Geometry check sheet. Reference: the model listing, model coordinates, mm. Give positions to 0.01 mm unless a question says otherwise; leave off trailing zeros. Write each loop counter-clockwise with the first axis right and the second up, starting at its lowest first coordinate (ties: lowest second). Pieces come first, ordered by that corner, then holes. Notation, with made-up numbers: (-22.75, -0.5) -> (28.25, -0.5) arc R16 ccw to (28.25, 15.5) -> close; hole circle Ø9 at (8, 40.5). An arc over 180 degrees is marked (long way). Write item = value, one per line. Start each with the question number.
1. Depth check by flat-ended pin: P1, Ø6, axis at x = -72.07, y = -115.97, coming from the -Z side; P2, Ø2.5, axis at x = 67.42, y = 66.68, coming from the -Z side; P3, Ø1.2, axis at y = -100.5, z = 44.5, coming from the -X side. Enter the tip coordinate at first touch or a pass-through.
2. Thickness scan on line 1 along Y through (x, z) = (16.5, 43.9) (3 decimals); line 2 along X through (y, z) = (115, 44.25); line 3 along X through (y, z) = (-67.5, 44.95). Record the ranges inside material, lowest first.
3. Cross-section at C-C, the plane z = 44.15. State how many separate pieces and enclosed holes the cut face has, plus the area to 3 significant figures.
4. Cross-section at A-A, the plane y = -13. Record the cut outline in (x, z).
5. Cross-section at D-D, the plane y = -44. Record the cut outline in (x, z), plus the area to 3 significant figures.
6. Cross-section at B-B, the plane x = -131. Record the cut outline in (y, z).
```python
from build123d import *

# Parameters (mm, degrees)
SKETCH_R        = 2.3622
SKETCH_R_2      = 17.78
PAD_DEPTH       = 2.3622
FILLET_R        = 6.35
FILLET001_R     = 6.35
FILLET002_R     = 6.35
FILLET003_R     = 6.35
FILLET004_R     = 6.35
FILLET005_R     = 3.175
FILLET006_R     = 3.175
FILLET007_R     = 6.35
FILLET008_R     = 6.35
FILLET009_R     = 6.35
FILLET010_R     = 6.35
FILLET011_R     = 6.35
FILLET012_R     = 3.175
FILLET013_R     = 3.175
SKETCH001_R     = 4.79425
POCKET_DEPTH    = 2.3632
SKETCH002_R     = 2.2479
POCKET001_DEPTH = 2.3632
SKETCH003_R     = 2.2479
POCKET002_DEPTH = 4.99999


with BuildPart() as part:
    # Sketch (on DatumPlane) → Pad (new body)
    with BuildSketch(Plane.XY.offset(43.6758)):
        Polygon((40.4368, 73.025), (-40.4368, 73.025), (-40.4368, 127), (-65.8368, 127), (-197.6882, 22.225), (-197.6882, -22.225), (-65.8368, -127), (-40.4368, -127), (-40.4368, -73.025), (40.4368, -73.025), (40.4368, -127), (72.1868, -127), (72.1868, 127), (40.4368, 127), align=None)
        with Locations((-21.3868, 66.675)):
            Circle(SKETCH_R, mode=Mode.SUBTRACT)
        with Locations((-21.3868, 53.975)):
            Circle(SKETCH_R, mode=Mode.SUBTRACT)
        with Locations((-21.3868, -53.975)):
            Circle(SKETCH_R, mode=Mode.SUBTRACT)
        with Locations((-21.3868, -66.675)):
            Circle(SKETCH_R, mode=Mode.SUBTRACT)
        with Locations((15.0368, 66.675)):
            Circle(SKETCH_R, mode=Mode.SUBTRACT)
        with Locations((15.24, 53.975)):
            Circle(SKETCH_R, mode=Mode.SUBTRACT)
        with Locations((15.24, -53.975)):
            Circle(SKETCH_R, mode=Mode.SUBTRACT)
        with Locations((15.24, -66.675)):
            Circle(SKETCH_R, mode=Mode.SUBTRACT)
        with Locations((-165.9382, 0)):
            Circle(SKETCH_R_2, mode=Mode.SUBTRACT)
    extrude(amount=PAD_DEPTH)

    # Fillet
    fillet_edges = [part.edges().sort_by_distance(p)[0] for p in [
        (-197.6882, -22.225, 44.8569),
    ]]
    fillet(fillet_edges, radius=FILLET_R)

    # Fillet001
    fillet001_edges = [part.edges().sort_by_distance(p)[0] for p in [
        (-65.8368, -127, 44.8569),
    ]]
    fillet(fillet001_edges, radius=FILLET001_R)

    # Fillet002
    fillet002_edges = [part.edges().sort_by_distance(p)[0] for p in [
        (-40.4368, -127, 44.8569),
    ]]
    fillet(fillet002_edges, radius=FILLET002_R)

    # Fillet003
    fillet003_edges = [part.edges().sort_by_distance(p)[0] for p in [
        (-40.4368, -73.025, 44.8569),
    ]]
    fillet(fillet003_edges, radius=FILLET003_R)

    # Fillet004
    fillet004_edges = [part.edges().sort_by_distance(p)[0] for p in [
        (40.4368, -73.025, 44.8569),
    ]]
    fillet(fillet004_edges, radius=FILLET004_R)

    # Fillet005
    fillet005_edges = [part.edges().sort_by_distance(p)[0] for p in [
        (40.4368, -127, 44.8569),
    ]]
    fillet(fillet005_edges, radius=FILLET005_R)

    # Fillet006
    fillet006_edges = [part.edges().sort_by_distance(p)[0] for p in [
        (72.1868, -127, 44.8569),
    ]]
    fillet(fillet006_edges, radius=FILLET006_R)

    # Fillet007
    fillet007_edges = [part.edges().sort_by_distance(p)[0] for p in [
        (-197.6882, 22.225, 44.8569),
    ]]
    fillet(fillet007_edges, radius=FILLET007_R)

    # Fillet008
    fillet008_edges = [part.edges().sort_by_distance(p)[0] for p in [
        (-65.8368, 127, 44.8569),
    ]]
    fillet(fillet008_edges, radius=FILLET008_R)

    # Fillet009
    fillet009_edges = [part.edges().sort_by_distance(p)[0] for p in [
        (-40.4368, 127, 44.8569),
    ]]
    fillet(fillet009_edges, radius=FILLET009_R)

    # Fillet010
    fillet010_edges = [part.edges().sort_by_distance(p)[0] for p in [
        (40.4368, 73.025, 44.8569),
    ]]
    fillet(fillet010_edges, radius=FILLET010_R)

    # Fillet011
    fillet011_edges = [part.edges().sort_by_distance(p)[0] for p in [
        (-40.4368, 73.025, 44.8569),
    ]]
    fillet(fillet011_edges, radius=FILLET011_R)

    # Fillet012
    fillet012_edges = [part.edges().sort_by_distance(p)[0] for p in [
        (40.4368, 127, 44.8569),
    ]]
    fillet(fillet012_edges, radius=FILLET012_R)

    # Fillet013
    fillet013_edges = [part.edges().sort_by_distance(p)[0] for p in [
        (72.1868, 127, 44.8569),
    ]]
    fillet(fillet013_edges, radius=FILLET013_R)

    # Sketch001 (on Face39 of Fillet013) → Pocket (cut, through all)
    with BuildSketch(Plane.XY.offset(46.038)):
        with Locations((-26.2382, 0)):
            Circle(SKETCH001_R)
    extrude(amount=-POCKET_DEPTH, mode=Mode.SUBTRACT)

    # Sketch002 (on Face44 of Pocket) → Pocket001 (cut, through all)
    with BuildSketch(Plane.XY.offset(46.038)):
        with Locations((-96.923253, -96.214243)):
            Circle(SKETCH002_R)
        with Locations((-72.065864, -115.967033)):
            Circle(SKETCH002_R)
        with Locations((-72.065864, 115.967033)):
            Circle(SKETCH002_R)
        with Locations((-96.923253, 96.214243)):
            Circle(SKETCH002_R)
    extrude(amount=-POCKET001_DEPTH, mode=Mode.SUBTRACT)

    # Sketch003 (on Face48 of Pocket001) → Pocket002 (cut)
    with BuildSketch(Plane.XY.offset(46.038)):
        with Locations((67.4243, -117.475)):
            Circle(SKETCH003_R)
        with Locations((67.4243, -66.675)):
            Circle(SKETCH003_R)
        with Locations((67.4243, 117.475)):
            Circle(SKETCH003_R)
        with Locations((67.4243, 66.675)):
            Circle(SKETCH003_R)
        with Locations((-177.3809, 19.819338)):
            Circle(SKETCH003_R)
        with Locations((-177.3809, -19.819338)):
            Circle(SKETCH003_R)
        with Locations((-143.0528, 0)):
            Circle(SKETCH003_R)
    extrude(amount=-POCKET002_DEPTH, mode=Mode.SUBTRACT)


solid = part.part
```
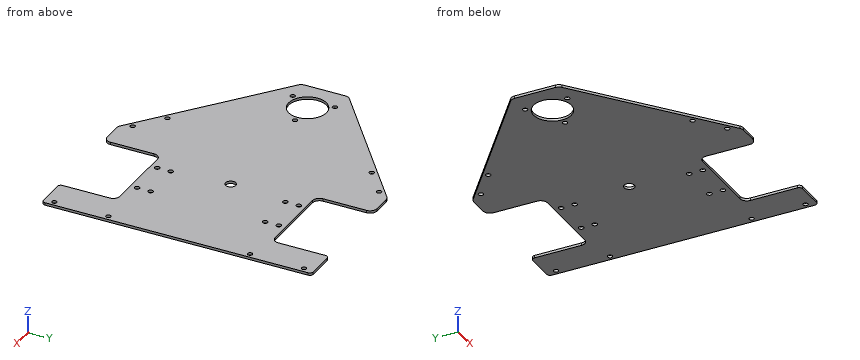
Answers:
q1.P1 = 43.68
q1.P2 = through
q1.P3 = -99.94
q2.line_1 = -73.025 to -68.673, -64.677 to -55.973, -51.977 to 51.977, 55.973 to 64.821, 68.529 to 73.025
q2.line_2 = -80.94 to -74.1, -70.04 to -40.44, 40.44 to 72.19
q2.line_3 = -140.71 to -23.6, -19.17 to 13.03, 17.45 to 65.33, 69.52 to 72.19
q3.separate_pieces = 1
q3.enclosed_holes = 21
q3.area = 44,600 mm^2
q4.outline = (-197.69, 43.68) -> (-178.07, 43.68) -> (-178.07, 46.04) -> (-197.69, 46.04) -> close; (-153.81, 43.68) -> (72.19, 43.68) -> (72.19, 46.04) -> (-153.81, 46.04) -> close
q5.outline = (-170.29, 43.68) -> (72.19, 43.68) -> (72.19, 46.04) -> (-170.29, 46.04) -> close
q5.area = 573 mm^2
q6.outline = (-75.22, 43.68) -> (75.22, 43.68) -> (75.22, 46.04) -> (-75.22, 46.04) -> close
